Can you work these out from the model? Positions are in its coordinate system, mm. Face numbers are marked on the shaded views. A direction names the side the tool comes from. Give positions to 0.01 mm unless a question says otherwise; leave off trailing zeros. Loops run counter-clockwise (first coordinate to the right, second up) from the corner with the lowest first, then second, coordinate; pieces in that order, holes last. Notation, with made-up numbers: (13.25, -13.75) -> (33.25, -13.75) arc R27 cw to (33.25, 22.25) -> close; hole circle Ø5 at (51, 19). An arc over 180 degrees is marked (long way). Use CSV: the item, a comma, the result in double quotes.
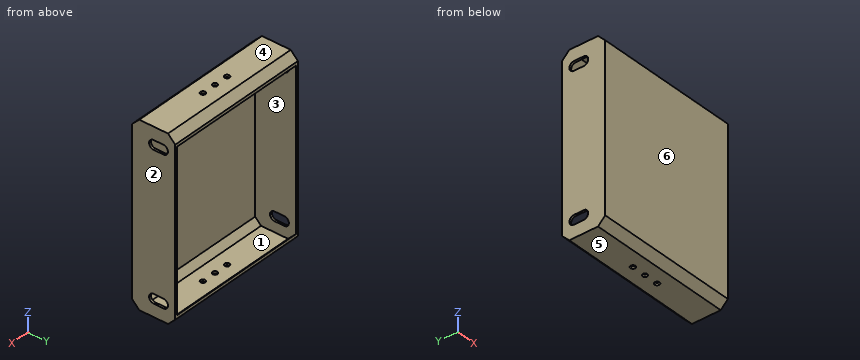
from build123d import *

# Parameters (mm, degrees)
SKETCH1_W                                = 203.2
SKETCH1_H                                = 247.65
BOSS_EXTRUDE1_DEPTH                      = 60
CHAMFER1_SIZE                            = 10
SHELL3_T                                 = -3
CUT_EXTRUDE1_REACH                       = 247.403
MIRROR1_AT_THE_SECOND_PLANE_COPY_1_REACH = 247.403
CUT_EXTRUDE2_REACH                       = 276.323
SKETCH3_R                                = 3.45


with BuildPart() as part:
    # Sketch1 → Boss-Extrude1 (new body)
    with BuildSketch(Plane(origin=(0, 0, 0), x_dir=(1, 0, 0), z_dir=(0, 1, 0))):
        Rectangle(SKETCH1_W, SKETCH1_H)
    extrude(amount=BOSS_EXTRUDE1_DEPTH)

    # Chamfer1
    chamfer1_edges = [part.edges().sort_by_distance(p)[0] for p in [
        (0, 60, 123.825),
        (0, 0, 123.825),
        (0, 0, -123.825),
        (0, 60, -123.825),
    ]]
    chamfer(chamfer1_edges, length=CHAMFER1_SIZE)

    # Shell3
    shell3_openings = [part.faces().sort_by_distance(p)[0] for p in [
        (0, 60, 0),
    ]]
    offset(amount=SHELL3_T, openings=shell3_openings, kind=Kind.INTERSECTION)

    # Sketch2 → Cut-Extrude1 (cut, up to next)
    with BuildSketch(Plane.ZY.offset(101.6), mode=Mode.PRIVATE) as cut_extrude1_sk1:
        with BuildLine():
            Line((-93.675, 43.55), (-93.675, 30))
            ThreePointArc((-93.675, 30), (-100.025, 23.65), (-106.375, 30))
            Line((-106.375, 30), (-106.375, 43.55))
            ThreePointArc((-106.375, 43.55), (-100.025, 49.9), (-93.675, 43.55))
        make_face()
    cut_extrude1_tool1 = extrude(cut_extrude1_sk1.sketch, amount=-CUT_EXTRUDE1_REACH, mode=Mode.PRIVATE) & part.part
    cut_extrude1 = cut_extrude1_tool1.solids().sort_by_distance((-101.6, 36.775, -100.025))[0]
    add(cut_extrude1, mode=Mode.SUBTRACT)

    # Mirror1: Cut-Extrude1 across plane
    add(cut_extrude1.mirror(Plane.XY), mode=Mode.SUBTRACT)

    # Mirror1 at the second plane: Cut-Extrude1 across plane
    add(cut_extrude1.mirror(Plane(origin=(0, 0, 0), x_dir=(0, 0, 1), z_dir=(1, 0, 0))), mode=Mode.SUBTRACT)

    # Mirror1 at the second plane copy 1 sketc → Mirror1 at the second plane copy 1 (cut, up to next)
    with BuildSketch(Plane(origin=(101.6, 0, 0), x_dir=(0, 0, -1), z_dir=(1, 0, 0)), mode=Mode.PRIVATE) as mirror1_at_the_second_plane_copy_1_sk1:
        with BuildLine():
            Line((-93.675, 43.55), (-93.675, 30))
            ThreePointArc((-93.675, 30), (-100.025, 23.65), (-106.375, 30))
            Line((-106.375, 30), (-106.375, 43.55))
            ThreePointArc((-106.375, 43.55), (-100.025, 49.9), (-93.675, 43.55))
        make_face()
    mirror1_at_the_second_plane_copy_1_tool1 = extrude(mirror1_at_the_second_plane_copy_1_sk1.sketch, amount=-MIRROR1_AT_THE_SECOND_PLANE_COPY_1_REACH, mode=Mode.PRIVATE) & part.part
    add(mirror1_at_the_second_plane_copy_1_tool1.solids().sort_by_distance((101.6, 36.775, 100.025))[0], mode=Mode.SUBTRACT)

    # Sketch3 → Cut-Extrude2 (cut, up to next)
    with BuildSketch(Plane(origin=(0, 0, -123.825), x_dir=(-1, 0, 0), z_dir=(0, 0, -1)), mode=Mode.PRIVATE) as cut_extrude2_sk1:
        with Locations((0, 30)):
            Circle(SKETCH3_R)
    cut_extrude2_tool1 = extrude(cut_extrude2_sk1.sketch, amount=-CUT_EXTRUDE2_REACH, mode=Mode.PRIVATE) & part.part
    # Sketch3 → Cut-Extrude2 (cut, up to next)
    with BuildSketch(Plane(origin=(0, 0, -123.825), x_dir=(-1, 0, 0), z_dir=(0, 0, -1)), mode=Mode.PRIVATE) as cut_extrude2_sk2:
        with Locations((20, 30)):
            Circle(SKETCH3_R)
    cut_extrude2_tool2 = extrude(cut_extrude2_sk2.sketch, amount=-CUT_EXTRUDE2_REACH, mode=Mode.PRIVATE) & part.part
    # Sketch3 → Cut-Extrude2 (cut, up to next)
    with BuildSketch(Plane(origin=(0, 0, -123.825), x_dir=(-1, 0, 0), z_dir=(0, 0, -1)), mode=Mode.PRIVATE) as cut_extrude2_sk3:
        with Locations((-20, 30)):
            Circle(SKETCH3_R)
    cut_extrude2_tool3 = extrude(cut_extrude2_sk3.sketch, amount=-CUT_EXTRUDE2_REACH, mode=Mode.PRIVATE) & part.part
    cut_extrude2_1 = cut_extrude2_tool1.solids().sort_by_distance((0, 30, -123.825))[0]
    add(cut_extrude2_1, mode=Mode.SUBTRACT)
    cut_extrude2_2 = cut_extrude2_tool2.solids().sort_by_distance((-20, 30, -123.825))[0]
    add(cut_extrude2_2, mode=Mode.SUBTRACT)
    cut_extrude2_3 = cut_extrude2_tool3.solids().sort_by_distance((20, 30, -123.825))[0]
    add(cut_extrude2_3, mode=Mode.SUBTRACT)
    cut_extrude2 = cut_extrude2_1 + cut_extrude2_2 + cut_extrude2_3  # Cut-Extrude2 as one shape, for the pattern or mirror that repeats it

    # Mirror2: Cut-Extrude2 across plane
    add(cut_extrude2.mirror(Plane.XY), mode=Mode.SUBTRACT)


solid = part.part
(1) If we section it at B-B, the plane x = 20: Write out the boundary of the cut face in (y, z) (3 decimals), then the cut area to 3 significant figures.
Answer sheet:
outline,"(0, -113.825) -> (10, -123.825) -> (26.55, -123.825) -> (26.55, -120.825) -> (11.243, -120.825) -> (3, -112.582) -> (3, 112.582) -> (11.243, 120.825) -> (26.55, 120.825) -> (26.55, 123.825) -> (10, 123.825) -> (0, 113.825) -> close; (33.45, -123.825) -> (50, -123.825) -> (60, -113.825) -> (60, -109.582) -> (48.757, -120.825) -> (33.45, -120.825) -> close; (33.45, 120.825) -> (48.757, 120.825) -> (60, 109.582) -> (60, 113.825) -> (50, 123.825) -> (33.45, 123.825) -> close"
area,"1,040 mm2"
(2) Will this pin go through, and if not, where does the flat tip stop? pin 1 Ø4 at (x, y) = (20, 30) entering from -Z.
Answer sheet:
pin 1,"passes through"
(3) We'd pull the mould along Z, two halves only. Please class the marked faces 3, 4, 5 and 6: released by +Z, released by -Z, zero draft, split by the parting line, or undercut.
Answer sheet:
face 3,"undercut"
face 4,"released by +Z"
face 5,"released by -Z"
face 6,"zero draft"
(4) Which directions (+Z, -Z, +X, -X, +Y, -Y) give clear straight access to the entire face, cutting with the end or side of a thin tool? Please do the marked faces 1 and 2.
Answer sheet:
face 1,"none"
face 2,"+Z, -Z, +X, +Y, -Y"
(5) If I drill on L1, parallel to X at y = 31.5, z = 20.5; L2, parallel to Z at x = 68.5, y = 37 (3 decimals); L3, parallel to Y at x = -67.5, z = -61, over which ranges is the centre line in solid material (lowest first)? Write a range as from..to.
Answer sheet:
L1,"x = -101.6..-98.6, 98.6..101.6"
L2,"z = -123.825..-120.825, 120.825..123.825"
L3,"y = 0..3"
(6) If we section it at C-C, the plane z = 36.5: Write out the boundary of the cut face in (x, y).
Answer sheet:
outline,"(-101.6, 0) -> (101.6, 0) -> (101.6, 60) -> (98.6, 60) -> (98.6, 3) -> (-98.6, 3) -> (-98.6, 60) -> (-101.6, 60) -> close"
(7) If we section it at A-A, the plane y = 40.5: Write out the boundary of the cut face in (x, z) (3 decimals).
Answer sheet:
outline,"(-101.6, -123.825) -> (101.6, -123.825) -> (101.6, -106.375) -> (98.6, -106.375) -> (98.6, -120.825) -> (-98.6, -120.825) -> (-98.6, -106.375) -> (-101.6, -106.375) -> close; (-101.6, -93.675) -> (-98.6, -93.675) -> (-98.6, 93.675) -> (-101.6, 93.675) -> close; (-101.6, 106.375) -> (-98.6, 106.375) -> (-98.6, 120.825) -> (98.6, 120.825) -> (98.6, 106.375) -> (101.6, 106.375) -> (101.6, 123.825) -> (-101.6, 123.825) -> close; (98.6, -93.675) -> (101.6, -93.675) -> (101.6, 93.675) -> (98.6, 93.675) -> close"
